Build history of the part. All positions in model axes, mm. A direction names the side the tool comes from. Round coordinates to 2 decimals unless told otherwise and drop trailing zeros. Order: outer loops, then holes, each group sorted by start corner. A loop starts at its lowest first (then second) coordinate and runs counter-clockwise, first axis right, second up. Notation, with made-up numbers: M 23,-17.75 L 79,-17.75 A12 cw 79,-1.75 Z; hole C -25.5,-18.5 d1. An arc over 180 degrees is marked long. One line per item, written item: value. Start each with the question number.
Item 1: Band-saw the part on B-B, the plane y = 0. Write the cut outline in (x, z), then the cut area to 3 significant figures.
Item 2: Band-saw the part on C-C, the plane x = -114.3. Write the cut outline in (y, z), then the cut area to 3 significant figures.
Item 3: Band-saw the part on A-A, the plane x = 38.1. Write the cut outline in (y, z).
Item 4: Band-saw the part on D-D, the plane y = 10.75. Write the cut outline in (x, z), then the cut area to 3 significant figures.
Item 5: Tool access for faces 1 (the flat face through (-25.4, 0, -2)), 2 (the cylindrical face through (-46.981, -0.178, 35.633)), 3 (the flat face through (-50.8, 0, -27)): list every direction of +Z, -Z, +X, -X, +Y, -Y with a clear straight run to the whole face (end or side of a thin tool).
Item 6: Probe L1, parallel to X at y = 0, z = -25; L2, parallel to Y at x = 38.1, z = -33.5; L3, parallel to Z at x = 29.5, y = 8.5. List the from-to ranges inside material, lowest first.
Item 7: Pin check, flat tips, straight feed: pin 1 (10 mm diameter, centred on x = -114.3, z = 0, fed in from -Y); pin 2 (12.5 mm diameter, centred on x = -108, y = -5, fed in from +Z); pin 3 (14.5 mm diameter, centred on x = 38.1, y = 0, fed in from +Z); pin 4 (4.5 mm diameter, centred on y = -5, z = -2, fed in from +X). Stop position of each tip, or through.
Item 8: Two-plate mould, pull along Z, no slides. Class faces 4 (the cylindrical face through (-21.58, -0.18, -13.31)), 5 (the flat face through (-127, 0, 0)), 6 (the cylindrical face through (-54.42, -0.18, 16.52)): +Z half, -Z half, draft (parallel to the pull), parting line (faces both ways), or undercut.
```python
from build123d import *

# Parameters (mm, degrees)
F0_R     = 6.35
F1_DEPTH = 12.7
F2_R     = 6.35
F3_DEPTH = 25.4
F4_R     = 6.35
F5_DEPTH = 25.4
F6_SIZE  = 6.35


# Not quite as in the source:
# - a feature names something its author has since deleted; it is built from what else it names


with BuildPart() as f1:
    # F0 (on Front) → F1 (new body, symmetric)
    with BuildSketch(Plane.XZ):
        with BuildLine():
            Line((-127, -12.7), (-63.5, -12.7))
            ThreePointArc((-63.5, -12.7), (-54.5197438789, -16.4197438789), (-50.8, -25.4))
            Line((-50.8, -25.4), (-50.8, -29.6333387181))
            ThreePointArc((-50.8, -29.6333387181), (-47.0802561211, -38.6135948391), (-38.1, -42.3333387181))
            Line((-38.1, -42.3333387181), (50.8, -42.3333387181))
            Line((50.8, -42.3333387181), (50.8, -16.9333387181))
            Line((50.8, -16.9333387181), (-12.7, -16.9333387181))
            ThreePointArc((-12.7, -16.9333387181), (-21.6802561211, -13.2135948391), (-25.4, -4.2333387181))
            Line((-25.4, -4.2333387181), (-25.4, 1.1545434965))
            ThreePointArc((-25.4, 1.1545434965), (-21.6802561211, 10.1347996175), (-12.7, 13.8545434965))
            Line((-12.7, 13.8545434965), (50.8, 13.8545434965))
            Line((50.8, 13.8545434965), (50.8, 39.2545434965))
            Line((50.8, 39.2545434965), (-38.1, 39.2545434965))
            ThreePointArc((-38.1, 39.2545434965), (-47.0802561211, 35.5347996175), (-50.8, 26.5545434965))
            Line((-50.8, 26.5545434965), (-50.8, 25.4))
            ThreePointArc((-50.8, 25.4), (-54.5197438789, 16.4197438789), (-63.5, 12.7))
            Line((-63.5, 12.7), (-127, 12.7))
            Line((-127, 12.7), (-127, -12.7))
        make_face()
        with Locations((-114.3, 0)):
            Circle(F0_R, mode=Mode.SUBTRACT)
    extrude(amount=F1_DEPTH, both=True)

    # F2 (on face) → F3 (cut)
    with BuildSketch(Plane(origin=(0, 0, 13.8545434965), x_dir=(1, 0, 0), z_dir=(0, 0, -1))):
        with Locations((38.1, 0)):
            Circle(F2_R)
    extrude(amount=-F3_DEPTH, mode=Mode.SUBTRACT)

    # F4 (on face) → F5 (cut)
    with BuildSketch(Plane(origin=(0, 0, -42.3333387181), x_dir=(1, 0, 0), z_dir=(0, 0, -1))):
        with Locations((38.1, 0)):
            Circle(F4_R)
    extrude(amount=-F5_DEPTH, mode=Mode.SUBTRACT)

    # F6
    f6_edges = [f1.edges().sort_by_distance(p)[0] for p in [
        (50.8, -12.7, -29.633339),
        (50.8, 12.7, -29.633339),
        (50.8, -12.7, 26.554543),
        (50.8, 12.7, 26.554543),
    ]]
    chamfer(f6_edges, length=F6_SIZE)


solid = f1.part
```
Output:
1. outline: M -127,-12.7 L -63.5,-12.7 A12.7 cw -50.8,-25.4 L -50.8,-29.63 A12.7 ccw -38.1,-42.33 L 31.75,-42.33 L 31.75,-16.93 L -12.7,-16.93 A12.7 cw -25.4,-4.23 L -25.4,1.15 A12.7 cw -12.7,13.85 L 31.75,13.85 L 31.75,39.25 L -38.1,39.25 A12.7 ccw -50.8,26.55 L -50.8,25.4 A12.7 cw -63.5,12.7 L -127,12.7 Z; M 44.45,-42.33 L 50.8,-42.33 L 50.8,-16.93 L 44.45,-16.93 Z; M 44.45,13.85 L 50.8,13.85 L 50.8,39.25 L 44.45,39.25 Z; hole C -114.3,0 d12.7
1. area: 7,180 mm²
2. outline: M -12.7,-12.7 L 12.7,-12.7 L 12.7,-6.35 L -12.7,-6.35 Z; M -12.7,6.35 L 12.7,6.35 L 12.7,12.7 L -12.7,12.7 Z
2. area: 323 mm²
3. outline: M -12.7,-42.33 L -6.35,-42.33 L -6.35,-16.93 L -12.7,-16.93 Z; M -12.7,13.85 L -6.35,13.85 L -6.35,39.25 L -12.7,39.25 Z; M 6.35,-42.33 L 12.7,-42.33 L 12.7,-16.93 L 6.35,-16.93 Z; M 6.35,13.85 L 12.7,13.85 L 12.7,39.25 L 6.35,39.25 Z
4. outline: M -127,-12.7 L -63.5,-12.7 A12.7 cw -50.8,-25.4 L -50.8,-29.63 A12.7 ccw -38.1,-42.33 L 46.4,-42.33 L 46.4,-16.93 L -12.7,-16.93 A12.7 cw -25.4,-4.23 L -25.4,1.15 A12.7 cw -12.7,13.85 L 46.4,13.85 L 46.4,39.25 L -38.1,39.25 A12.7 ccw -50.8,26.55 L -50.8,25.4 A12.7 cw -63.5,12.7 L -127,12.7 Z; hole C -114.3,0 d12.7
4. area: 7,600 mm²
5. face 1: +X, +Y, -Y
5. face 2: +Z, -X, +Y, -Y
5. face 3: -Z, -X, +Y, -Y
6. L1: x = -50.81 to 31.75, 44.45 to 50.8
6. L2: y = -12.7 to -6.35, 6.35 to 12.7
6. L3: z = -42.33 to -16.93, 13.85 to 39.25
7. pin 1: passes through
7. pin 2: stops at z = 12.7
7. pin 3: stops at z = 39.25
7. pin 4: stops at x = -25.4
8. face 4: undercut
8. face 5: draft
8. face 6: +Z half
